```python
from build123d import *

# Parameters (mm, degrees)
ESBO_O1_R                = 1.85525586
RESSALTO_EXTRUS_O1_DEPTH = 19
CORTE_EXTRUS_O1_DEPTH    = 18
ESBO_O3_R                = 2.5
RESSALTO_EXTRUS_O2_DEPTH = 7


with BuildPart() as part:
    # Esboço1 → Ressalto-extrusão1 (new body)
    with BuildSketch(Plane.XY):
        with BuildLine():
            Line((17.75, 3.5), (12.410650194, 3.5))
            ThreePointArc((12.410650194, 3.5), (0, 12.894736842), (-12.410650194, 3.5))
            Line((-12.410650194, 3.5), (-17.75, 3.5))
            ThreePointArc((-17.75, 3.5), (-21.25, 0), (-17.75, -3.5))
            Line((-17.75, -3.5), (-12.410650194, -3.5))
            ThreePointArc((-12.410650194, -3.5), (-10.341581818, -7.702332356), (-6.907894737, -10.888306964))
            Line((-6.907894737, -10.888306964), (-6.907894737, -12.894736842))
            Line((-6.907894737, -12.894736842), (-6.907894737, -15.657894737))
            Line((-6.907894737, -15.657894737), (6.907894737, -15.657894737))
            Line((6.907894737, -15.657894737), (6.907894737, -12.894736842))
            Line((6.907894737, -12.894736842), (6.907894737, -10.888306964))
            ThreePointArc((6.907894737, -10.888306964), (10.341581818, -7.702332356), (12.410650194, -3.5))
            Line((12.410650194, -3.5), (17.75, -3.5))
            ThreePointArc((17.75, -3.5), (21.25, 0), (17.75, 3.5))
        make_face()
        with Locations((17.75, 0)):
            Circle(ESBO_O1_R, mode=Mode.SUBTRACT)
        with Locations((-17.75, 0)):
            Circle(ESBO_O1_R, mode=Mode.SUBTRACT)
    extrude(amount=RESSALTO_EXTRUS_O1_DEPTH)

    # Esboço2 → Corte-extrusão1 (cut)
    with BuildSketch(Plane(origin=(0, 0, 0), x_dir=(-1, 0, 0), z_dir=(0, 0, -1))):
        with BuildLine():
            Line((12.410650194, 3.5), (23.80699558, 3.5))
            Line((23.80699558, 3.5), (23.80699558, -3.5))
            Line((23.80699558, -3.5), (12.410650194, -3.5))
            ThreePointArc((12.410650194, -3.5), (12.894736842, 0), (12.410650194, 3.5))
        make_face()
        with BuildLine():
            Line((-12.410650194, 3.5), (-24.760546325, 3.5))
            Line((-24.760546325, 3.5), (-24.760546325, -3.5))
            Line((-24.760546325, -3.5), (-12.410650194, -3.5))
            ThreePointArc((-12.410650194, -3.5), (-12.894736842, 0), (-12.410650194, 3.5))
        make_face()
    extrude(amount=-CORTE_EXTRUS_O1_DEPTH, mode=Mode.SUBTRACT)

    # Esboço3 → Ressalto-extrusão2 (add)
    with BuildSketch(Plane.XY.offset(19)):
        with Locations((0, 6.5)):
            Circle(ESBO_O3_R)
    extrude(amount=RESSALTO_EXTRUS_O2_DEPTH)


solid = part.part
```
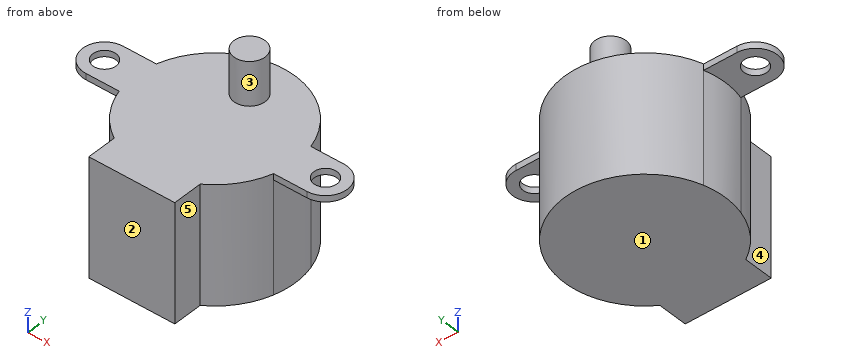
Work out the finished part from the listing and answer in its coordinate system (mm). Face numbers are marked on the shaded views. A direction names the side the tool comes from. Coordinates: 2 decimals unless noted, no trailing zeros. Loops run counter-clockwise (first coordinate to the right, second up) from the corner with the lowest first, then second, coordinate; pieces in that order, holes last. Notation, with made-up numbers: M -29.5,-8 L -15.5,-8 A9 cw -15.5,5 Z; hole C 19,-0.75 d8. An arc over 180 degrees is marked long. Use CSV: the item, a comma, the result in double quotes. Start each with the question number.
(1) Find section D-D, the plane x = 0. Give the vertices of the cut face in (y, z).
(2) Consider line 1 (X direction, y = 0, z = 18.7); line 2 (Y direction, x = 17.75, z = 18.5); line 3 (Z direction, x = -4, y = 8). Determine where each line is inside the solid, lowest interval first.
(3) For the marked faces 1, 2, 3, 4 and 5, determine the directions among +Z, -Z, +X, -X, +Y, -Y from which every point of the face is accessible in a straight line to the end or side of a thin tool.
(4) Find section C-C, the plane z = 6.25. Give the vertices of the cut face in (x, y), then the cut area to 3 significant figures.
(5) Given pin 1 Ø3 at (y, z) = (-7, 5) entering from +X; pin 2 Ø5.5 at (x, y) = (18, -0.5) entering from -Z; pin 3 Ø5 at (y, z) = (-8, 19.5) entering from +X; pin 4 Ø2 at (x, y) = (-17.5, -0.5) entering from -Z, each flat-ended and moving along its own axis, determine where each tip first touches the part or whether it passes through.
(6) Find section B-B, the plane x = 19. Give the vertices of the cut face in (y, z).
(7) Find section A-A, the plane y = 0. Give the vertices of the cut face in (x, z).
Recorded:
1,outline,"M -15.66,0 L 12.89,0 L 12.89,19 L 9,19 L 9,26 L 4,26 L 4,19 L -15.66,19 Z"
2,line 1,"x = -21.25 to -19.61, -15.89 to 15.89, 19.61 to 21.25"
2,line 2,"y = -3.5 to -1.86, 1.86 to 3.5"
2,line 3,"z = 0 to 19"
3,face 1,"-Z, +X, -X, +Y, -Y"
3,face 2,"+Z, -Z, +X, -X, -Y"
3,face 3,"+Z"
3,face 4,"+Z, -Z, -X, -Y"
3,face 5,"+Z, -Z, +X, -Y"
4,outline,"M -6.91,-15.66 L 6.91,-15.66 L 6.91,-10.89 A12.89 ccw long -6.91,-10.89 Z"
4,area,"569 mm^2"
5,pin 1,"stops at x = 11.66"
5,pin 2,"stops at z = 18"
5,pin 3,"stops at x = 11.64"
5,pin 4,"passes through"
6,outline,"M -3.27,18 L -1.37,18 L -1.37,19 L -3.27,19 Z; M 1.37,18 L 3.27,18 L 3.27,19 L 1.37,19 Z"
7,outline,"M -21.25,18 L -19.61,18 L -19.61,19 L -21.25,19 Z; M -15.89,18 L -12.89,18 L -12.89,0 L 12.89,0 L 12.89,18 L 15.89,18 L 15.89,19 L -15.89,19 Z; M 19.61,18 L 21.25,18 L 21.25,19 L 19.61,19 Z"
